Could you check a few things on this model? Use its own coordinates, in mm. Face numbers are marked on the shaded views. A direction names the side the tool comes from. Coordinates: 2 decimals unless noted, no trailing zeros. Write each loop counter-clockwise with the first axis right and the second up, starting at its lowest first coordinate (ties: lowest second). Pieces come first, ordered by that corner, then holes.
```python
from build123d import *

# Parameters (mm, degrees)
BOSS_EXTRUDE2_DEPTH = 60
BOSS_EXTRUDE3_DEPTH = 10
CUT_EXTRUDE2_REACH  = 97.673
SKETCH8_R           = 4.75
SKETCH8_R_2         = 3
CUT_EXTRUDE3_REACH  = 87
SKETCH9_R           = 7.5
CUT_EXTRUDE4_REACH  = 87
SKETCH10_R          = 7
SKETCH12_R          = 7.5
CUT_EXTRUDE6_DEPTH  = 10
CUT_EXTRUDE16_REACH = 52
SKETCH24_R          = 2.25
SKETCH33_R          = 1.5
CUT_EXTRUDE18_DEPTH = 10
SKETCH37_W          = 85
SKETCH37_H          = 60
BOSS_EXTRUDE7_DEPTH = 5
SKETCH38_R          = 2.5
SKETCH38_R_2        = 2
CUT_EXTRUDE19_DEPTH = 20
CUT_EXTRUDE20_REACH = 87
SKETCH39_R          = 2.5
SKETCH40_R          = 2
CUT_EXTRUDE21_DEPTH = 10
SKETCH41_R          = 1.15
CUT_EXTRUDE22_DEPTH = 2.5


with BuildPart() as part:
    # Sketch1 → Boss-Extrude2 (new body)
    with BuildSketch(Plane(origin=(0, 0, 0), x_dir=(1, 0, 0), z_dir=(0, 1, 0))):
        Polygon((-42.705817414, 39.602616449), (-42.705817414, -40.397383551), (42.294182586, -40.397383551), (42.294182586, 9.904131639), (12.595697776, 39.602616449), align=None)
        Polygon((-17.705817414, 28.992616449), (-17.705817414, -29.787383551), (31.69097915, -29.787383551), (31.69097915, -0.705868361), (1.992494341, 28.992616449), align=None, mode=Mode.SUBTRACT)
    extrude(amount=BOSS_EXTRUDE2_DEPTH)

    # Sketch4 → Boss-Extrude3 (add)
    with BuildSketch(Plane(origin=(0, 0, 0), x_dir=(-1, 0, 0), z_dir=(0, -1, 0))):
        Polygon((17.705817414, 28.992616449), (-1.992494341, 28.992616449), (-31.69097915, -0.705868361), (-31.69097915, -29.787383551), (17.705817414, -29.787383551), align=None)
    extrude(amount=-BOSS_EXTRUDE3_DEPTH)

    # Sketch8 → Cut-Extrude2 (cut, up to next)
    with BuildSketch(Plane(origin=(26.099157113, 0, -26.099157113), x_dir=(-0.707106781, 0, -0.707106781), z_dir=(0.707106781, 0, -0.707106781)), mode=Mode.PRIVATE) as cut_extrude2_sk1:
        with Locations((11.096775332, 48)):
            Circle(SKETCH8_R)
    cut_extrude2_tool1 = extrude(cut_extrude2_sk1.sketch, amount=-CUT_EXTRUDE2_REACH, mode=Mode.PRIVATE) & part.part
    add(cut_extrude2_tool1.solids().sort_by_distance((18.252552, 48, -33.945762))[0], mode=Mode.SUBTRACT)
    # Sketch8 → Cut-Extrude2 (cut, up to next)
    with BuildSketch(Plane(origin=(26.099157113, 0, -26.099157113), x_dir=(-0.707106781, 0, -0.707106781), z_dir=(0.707106781, 0, -0.707106781)), mode=Mode.PRIVATE) as cut_extrude2_sk2:
        with Locations((11.096775332, 34)):
            Circle(SKETCH8_R_2)
    cut_extrude2_tool2 = extrude(cut_extrude2_sk2.sketch, amount=-CUT_EXTRUDE2_REACH, mode=Mode.PRIVATE) & part.part
    add(cut_extrude2_tool2.solids().sort_by_distance((18.252552, 34, -33.945762))[0], mode=Mode.SUBTRACT)
    # Sketch8 → Cut-Extrude2 (cut, up to next)
    with BuildSketch(Plane(origin=(26.099157113, 0, -26.099157113), x_dir=(-0.707106781, 0, -0.707106781), z_dir=(0.707106781, 0, -0.707106781)), mode=Mode.PRIVATE) as cut_extrude2_sk3:
        with Locations((11.096775332, 22)):
            Circle(SKETCH8_R)
    cut_extrude2_tool3 = extrude(cut_extrude2_sk3.sketch, amount=-CUT_EXTRUDE2_REACH, mode=Mode.PRIVATE) & part.part
    add(cut_extrude2_tool3.solids().sort_by_distance((18.252552, 22, -33.945762))[0], mode=Mode.SUBTRACT)
    # Sketch8 → Cut-Extrude2 (cut, up to next)
    with BuildSketch(Plane(origin=(26.099157113, 0, -26.099157113), x_dir=(-0.707106781, 0, -0.707106781), z_dir=(0.707106781, 0, -0.707106781)), mode=Mode.PRIVATE) as cut_extrude2_sk4:
        with Locations((-0.903224668, 22)):
            Circle(SKETCH8_R_2)
    cut_extrude2_tool4 = extrude(cut_extrude2_sk4.sketch, amount=-CUT_EXTRUDE2_REACH, mode=Mode.PRIVATE) & part.part
    add(cut_extrude2_tool4.solids().sort_by_distance((26.737833, 22, -25.460481))[0], mode=Mode.SUBTRACT)
    # Sketch8 → Cut-Extrude2 (cut, up to next)
    with BuildSketch(Plane(origin=(26.099157113, 0, -26.099157113), x_dir=(-0.707106781, 0, -0.707106781), z_dir=(0.707106781, 0, -0.707106781)), mode=Mode.PRIVATE) as cut_extrude2_sk5:
        with Locations((-14.903224668, 22)):
            Circle(SKETCH8_R)
    cut_extrude2_tool5 = extrude(cut_extrude2_sk5.sketch, amount=-CUT_EXTRUDE2_REACH, mode=Mode.PRIVATE) & part.part
    add(cut_extrude2_tool5.solids().sort_by_distance((36.637328, 22, -15.560986))[0], mode=Mode.SUBTRACT)

    # Sketch9 → Cut-Extrude3 (cut, up to next)
    with BuildSketch(Plane.ZY.offset(42.705817414), mode=Mode.PRIVATE) as cut_extrude3_sk1:
        with Locations((-4.602616449, 35)):
            Circle(SKETCH9_R)
    cut_extrude3_tool1 = extrude(cut_extrude3_sk1.sketch, amount=-CUT_EXTRUDE3_REACH, mode=Mode.PRIVATE) & part.part
    add(cut_extrude3_tool1.solids().sort_by_distance((-42.705817, 35, -4.602616))[0], mode=Mode.SUBTRACT)

    # Sketch10 → Cut-Extrude4 (cut, up to next)
    with BuildSketch(Plane(origin=(42.294182586, 0, 0), x_dir=(0, 0, -1), z_dir=(1, 0, 0)), mode=Mode.PRIVATE) as cut_extrude4_sk1:
        with Locations((-13.397383551, 35)):
            Circle(SKETCH10_R)
    cut_extrude4_tool1 = extrude(cut_extrude4_sk1.sketch, amount=-CUT_EXTRUDE4_REACH, mode=Mode.PRIVATE) & part.part
    add(cut_extrude4_tool1.solids().sort_by_distance((42.294183, 35, 13.397384))[0], mode=Mode.SUBTRACT)

    # Sketch12 → Cut-Extrude6 (cut)
    with BuildSketch(Plane(origin=(0, 60, 0), x_dir=(1, 0, 0), z_dir=(0, 1, 0))):
        with Locations((-30.205817414, 4.602616449)):
            Circle(SKETCH12_R)
    extrude(amount=-CUT_EXTRUDE6_DEPTH, mode=Mode.SUBTRACT)

    # Sketch24 → Cut-Extrude16 (cut, up to next)
    with BuildSketch(Plane(origin=(0, 50, 0), x_dir=(1, 0, 0), z_dir=(0, 1, 0)), mode=Mode.PRIVATE) as cut_extrude16_sk1:
        with Locations((-26.455817414, 4.602616449)):
            Circle(SKETCH24_R)
    cut_extrude16_tool1 = extrude(cut_extrude16_sk1.sketch, amount=-CUT_EXTRUDE16_REACH, mode=Mode.PRIVATE) & part.part
    add(cut_extrude16_tool1.solids().sort_by_distance((-26.455817, 50, -4.602616))[0], mode=Mode.SUBTRACT)
    # Sketch24 → Cut-Extrude16 (cut, up to next)
    with BuildSketch(Plane(origin=(0, 50, 0), x_dir=(1, 0, 0), z_dir=(0, 1, 0)), mode=Mode.PRIVATE) as cut_extrude16_sk2:
        with Locations((-33.955817414, 4.602616449)):
            Circle(SKETCH24_R)
    cut_extrude16_tool2 = extrude(cut_extrude16_sk2.sketch, amount=-CUT_EXTRUDE16_REACH, mode=Mode.PRIVATE) & part.part
    add(cut_extrude16_tool2.solids().sort_by_distance((-33.955817, 50, -4.602616))[0], mode=Mode.SUBTRACT)

    # Sketch33 → Cut-Extrude18 (cut)
    with BuildSketch(Plane.ZY.offset(42.705817414)):
        with Locations((5.397383551, 38)):
            Circle(SKETCH33_R)
        with Locations((5.397383551, 32)):
            Circle(SKETCH33_R)
    extrude(amount=-CUT_EXTRUDE18_DEPTH, mode=Mode.SUBTRACT)

    # Sketch37 → Boss-Extrude7 (add)
    with BuildSketch(Plane.XY.offset(40.397383551)):
        with Locations((-0.205817414, 30)):
            Rectangle(SKETCH37_W, SKETCH37_H)
    extrude(amount=BOSS_EXTRUDE7_DEPTH)

    # Sketch38 → Cut-Extrude19 (cut)
    with BuildSketch(Plane.ZY.offset(42.705817414)):
        with Locations((-19.602616449, 5)):
            Circle(SKETCH38_R)
        with Locations((25.397383551, 5)):
            Circle(SKETCH38_R)
        with Locations((-36.852616449, 40)):
            Circle(SKETCH38_R_2)
        with Locations((42.647383551, 40)):
            Circle(SKETCH38_R_2)
    extrude(amount=-CUT_EXTRUDE19_DEPTH, mode=Mode.SUBTRACT)

    # Sketch39 → Cut-Extrude20 (cut, up to next)
    with BuildSketch(Plane.ZY.offset(42.705817414), mode=Mode.PRIVATE) as cut_extrude20_sk1:
        with Locations((-14.602616449, 15)):
            Circle(SKETCH39_R)
    cut_extrude20_tool1 = extrude(cut_extrude20_sk1.sketch, amount=-CUT_EXTRUDE20_REACH, mode=Mode.PRIVATE) & part.part
    add(cut_extrude20_tool1.solids().sort_by_distance((-42.705817, 15, -14.602616))[0], mode=Mode.SUBTRACT)

    # Sketch40 → Cut-Extrude21 (cut)
    with BuildSketch(Plane.XZ):
        with Locations((-36.705817414, -33.602616449)):
            Circle(SKETCH40_R)
        with Locations((-36.705817414, 39.397383551)):
            Circle(SKETCH40_R)
        with Locations((36.294182586, 39.397383551)):
            Circle(SKETCH40_R)
        with Locations((36.294182586, -7.418850265)):
            Circle(SKETCH40_R)
        with Locations((10.110416402, -33.602616449)):
            Circle(SKETCH40_R)
    extrude(amount=-CUT_EXTRUDE21_DEPTH, mode=Mode.SUBTRACT)

    # Sketch41 → Cut-Extrude22 (cut)
    with BuildSketch(Plane(origin=(26.099157113, 0, -26.099157113), x_dir=(-0.707106781, 0, -0.707106781), z_dir=(0.707106781, 0, -0.707106781))):
        with Locations((14.096775332, 34)):
            Circle(SKETCH41_R)
        with Locations((8.096775332, 34)):
            Circle(SKETCH41_R)
        with Locations((-0.903224668, 25)):
            Circle(SKETCH41_R)
        with Locations((-0.903224668, 19)):
            Circle(SKETCH41_R)
    extrude(amount=-CUT_EXTRUDE22_DEPTH, mode=Mode.SUBTRACT)


solid = part.part
```
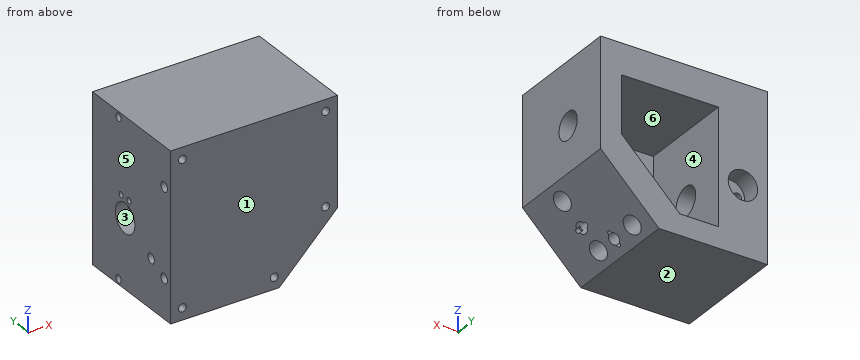
1. If we mould it in two halves opening along Z, with no side actions, what happens to the marked faces 1, 2, 3 and 4? For each: pulls with the +Z half, pulls with the -Z half, needs draft (parallel to the pull), parting line crosses it, or undercut.
Verdict:
face 1: needs draft
face 2: pulls with the -Z half
face 3: undercut
face 4: undercut
2. For pin 1 (3.5 mm diameter, centred on y = 32, z = 5.5, fed in from -X); pin 2 (5 mm diameter, centred on x = -26.46, z = -4.6, fed in from +Y); pin 3 (4.5 mm diameter, centred on y = 15, z = -14.6, fed in from -X); pin 4 (2 mm diameter, centred on x = 10.5, z = -33, fed in from -Y), each with a flat end and sliding along its axis, tell me the tip position at first contact or that it passes through.
Verdict:
pin 1: stops at x = -42.71
pin 2: stops at y = 50
pin 3: stops at x = 14.14
pin 4: stops at y = 10
3. I want a section at A-A on y = 15. Please give me the cut outline in (x, z), plus the area to 3 significant figures.
Verdict:
outline: (-42.71, -39.6) - (12.6, -39.6) - (42.29, -9.9) - (42.29, 45.4) - (-42.71, 45.4) - (-42.71, -12.1) - (-17.71, -12.1) - (-17.71, 29.79) - (31.69, 29.79) - (31.69, 0.71) - (1.99, -28.99) - (-17.71, -28.99) - (-17.71, -17.1) - (-42.71, -17.1) - close
area: 4,200 mm2
4. I want a section at D-D on x = -19.5. Please give me the cut outline in (y, z).
Verdict:
outline: (0, -39.6) - (60, -39.6) - (60, 45.4) - (0, 45.4) - close; hole circle Ø5 at (15, -14.6); hole circle Ø15 at (35, -4.6)
5. Please list where these lines run through material, in increasing order: line 1 along Z through (x, y) = (-2.5, 55.5); line 2 along X through (y, z) = (3, -34); line 3 along Z through (x, y) = (11, 12.5).
Verdict:
line 1: z = -39.6 to -28.99, 29.79 to 45.4
line 2: x = -42.71 to -38.67, -34.75 to 8.15, 12.07 to 18.2
line 3: z = -39.6 to -19.99, 29.79 to 45.4
6. I want a section at C-C on z = 14. Please give me the cut outline in (x, y).
Verdict:
outline: (-42.71, 0) - (42.29, 0) - (42.29, 28.03) - (31.69, 28.03) - (31.69, 10) - (-17.71, 10) - (-17.71, 60) - (-42.71, 60) - close; (31.69, 41.97) - (42.29, 41.97) - (42.29, 60) - (31.69, 60) - close
7. On a 3-axis mill with a long thin cutter (end or side, diameter ignored), from which of +Z, -Z, +X, -X, +Y, -Y can I reach the whole of each face in a straight line? I mean the marked faces 5 and 6. Say none if no direction works.
Verdict:
face 5: +Z, -Z, -X, +Y, -Y
face 6: +Y
8. I want a section at B-B on x = -4. Please give me the cut outline in (y, z).
Verdict:
outline: (0, -39.6) - (60, -39.6) - (60, -28.99) - (10, -28.99) - (10, 29.79) - (60, 29.79) - (60, 45.4) - (0, 45.4) - close
